Can you work these out from the drawing? Everything is in mm from the part's minimum corner. A direction names the side the tool comes from. Coordinates: 2 decimals unless noted, no trailing zeros. Loops run counter-clockwise (first coordinate to the right, second up) from the corner with the lowest first, then second, coordinate; pieces in that order, holes last. Notation, with made-up numbers: (71, 25) -> (86, 25) arc R30 cw to (86, 56) -> close; hole circle Ø2 at (5, 80.25). An arc over 180 degrees is marked (long way). Put each result on its own line as item: value. Start each with the question number.
Item 1: If we section it at B-B on y = 13: Please give me the cut outline in (x, z).
Item 2: If we section it at D-D on z = 36: Please give me the cut outline in (x, y), plus the area to 3 significant figures.
Item 3: Please list where these lines run through material, in increasing order: L1, parallel to X at y = 47.5, z = 34; L2, parallel to X at y = 39, z = 12; L3, parallel to Y at x = 7.5, z = 33. Write a range as from..to.
Item 4: Will these pins go through, and if not, where does the flat tip stop? P1, Ø9, axis at x = 86, z = 40.5, coming from the -Y side; P2, Ø22, axis at y = 15.5, z = 44, coming from the +X side; P3, Ø12, axis at x = 48.5, y = 36, coming from the -Z side.
Item 5: For the marked faces 4, 5, 6 and 7, which set-ups out of +Z, -Z, +X, -X, +Y, -Y let a thin tool reach every point of the face, with its end or its side?
Item 6: If we section it at A-A on z = 9: Please give me the cut outline in (x, y).
Item 7: We'd pull the mould along X, two halves only. Please class the marked faces 1, 2 and 3: pulls with the +X half, pulls with the -X half, needs draft (parallel to the pull), parting line crosses it, or undercut.
Item 8: If we section it at C-C on x = 13.5: Please give me the cut outline in (y, z).
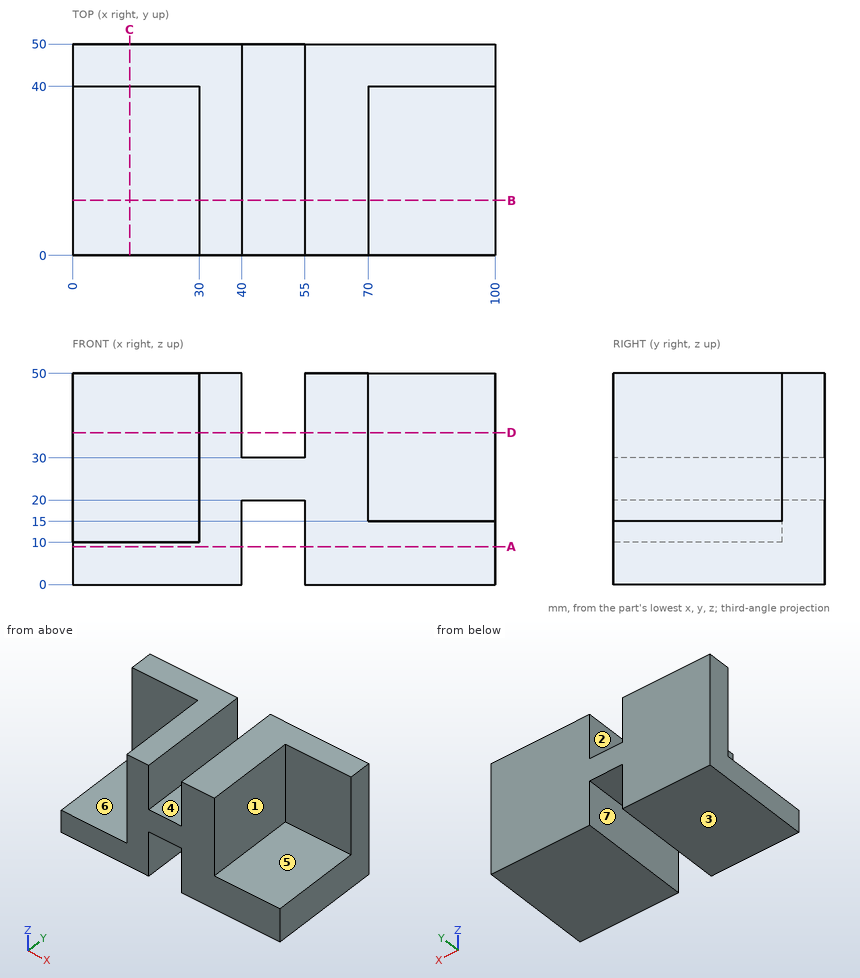
Solutions:
1. outline: (0, 0) -> (40, 0) -> (40, 20) -> (55, 20) -> (55, 0) -> (100, 0) -> (100, 15) -> (70, 15) -> (70, 50) -> (55, 50) -> (55, 30) -> (40, 30) -> (40, 50) -> (30, 50) -> (30, 10) -> (0, 10) -> close
2. outline: (0, 40) -> (30, 40) -> (30, 0) -> (40, 0) -> (40, 50) -> (0, 50) -> close; (55, 0) -> (70, 0) -> (70, 40) -> (100, 40) -> (100, 50) -> (55, 50) -> close
2. area: 1,850 mm^2
3. L1: 0..40, 55..100
3. L2: 30..40, 55..100
3. L3: 40..50
4. P1: y = 40
4. P2: x = 70
4. P3: z = 20
5. face 4: +Z, +Y, -Y
5. face 5: +Z, +X, -Y
5. face 6: +Z, -X, -Y
5. face 7: -Z, +Y, -Y
6. outline: (0, 0) -> (40, 0) -> (40, 50) -> (0, 50) -> close; (55, 0) -> (100, 0) -> (100, 50) -> (55, 50) -> close
7. face 1: pulls with the +X half
7. face 2: undercut
7. face 3: needs draft
8. outline: (0, 0) -> (50, 0) -> (50, 50) -> (40, 50) -> (40, 10) -> (0, 10) -> close
